Could you check a few things on this model? Use its own coordinates, in mm. A direction names the side the tool comes from. Coordinates: 2 decimals unless noted, no trailing zeros. Loops run counter-clockwise (first coordinate to the right, second up) from the corner with the lowest first, then second, coordinate; pieces in that order, holes last. Notation, with made-up numbers: (72, 25) -> (78, 25) arc R5 ccw to (78, 30) -> close; hole circle Ø2 at (42, 38). An arc over 180 degrees is marked (long way). One line per question, with ' | ' between items. Start each with the question number.
(1) Suppose I cut it at B-B (z = -14.5). Please give me the cut outline in (x, y).
(2) If we mould it in two halves opening along Z, with no side actions, what happens to faces 6 (the face through (0.27, -10.4, 43.93)), 7 (the face through (-12, -1, 26)), 8 (the face through (-9, 3.5, -45))? For each: pulls with the +Z half, pulls with the -Z half, needs draft (parallel to the pull), parting line crosses it, or undercut.
(3) Which directions (+Z, -Z, +X, -X, +Y, -Y) give clear straight access to the entire face, cutting with the end or side of a thin tool? Please do faces 1 (the face through (9.56, -6.07, 26.04)), 2 (the face through (-9, -1.5, -45)), 3 (the face through (0, 11, -1)), 4 (the face through (14.6, -7.2, -47)), 5 (the face through (-21, 0, 1)).
(4) Suppose I cut it at D-D (x = 1). Please give me the cut outline in (y, z), plus the area to 3 significant figures.
(5) Suppose I cut it at A-A (y = -6). Please give me the cut outline in (x, z), plus the area to 3 significant figures.
(6) If I drill on line 1 along X through (y, z) = (-6.5, 25.5); line 2 along X through (y, z) = (-7, -16.5); line 3 along Z through (x, y) = (-8, 8.75), over which ranges is the centre line in solid material (lowest first)?
(7) I'm going to push flat-ended pins straight in: pin 1 Ø4 at (x, y) = (-8, 0.5) entering from -Z; pin 2 Ø2.5 at (x, z) = (12, 25) entering from -Y; pin 3 Ø1 at (y, z) = (0, -45.5) entering from -X. Where does each tip first touch, or does it pass through?
(8) Suppose I cut it at C-C (y = 5). Please give me the cut outline in (x, z).
```python
from build123d import *

# Parameters (mm, degrees)
EXTRUDE_370_DEPTH      = 11
EXTRUDE_370_DEPTH_BACK = 11
SKETCH_1_W             = 42
SKETCH_1_H             = 89
SKETCH_2_W             = 7
SKETCH_2_H             = 5
EXTRUDE_597_DEPTH      = 2
SKETCH_3_R             = 2
EXTRUDE_827_DEPTH      = 5
SKETCH_4_R             = 2.5
CUT_EXTRUDE_1027_DEPTH = 10
FILLET_1_R             = 2


with BuildPart() as part:
    # Sketch 1 → Extrude 370 (new, two sides: drawn at the far end of the back side and taken through both)
    with BuildSketch(Plane(origin=(0, 0, 0), x_dir=(1, 0, 0), z_dir=(0, 1, 0)).offset(-EXTRUDE_370_DEPTH_BACK)):
        Rectangle(SKETCH_1_W, SKETCH_1_H)
    extrude(amount=EXTRUDE_370_DEPTH + EXTRUDE_370_DEPTH_BACK)

    # Sketch 2 → Extrude 597 (add)
    with BuildSketch(Plane(origin=(0, 0, -44.5), x_dir=(-1, 0, 0), z_dir=(0, 0, -1))):
        with Locations((9, 1)):
            Rectangle(SKETCH_2_W, SKETCH_2_H)
    extrude(amount=EXTRUDE_597_DEPTH)

    # Sketch 3 → Extrude 827 (add)
    with BuildSketch(Plane(origin=(0, 0, -44.5), x_dir=(-1, 0, 0), z_dir=(0, 0, -1))):
        with Locations((-13, -6)):
            Circle(SKETCH_3_R)
    extrude(amount=EXTRUDE_827_DEPTH)

    # Sketch 4 → Cut-Extrude 1027 (cut)
    with BuildSketch(Plane.XZ.offset(11)):
        with Locations(Location((-12, 25.5, 0), (0, 0, 270))):
            Circle(SKETCH_4_R)
        with Locations(Location((12, 25.5, 0), (0, 0, 270))):
            Circle(SKETCH_4_R)
        with Locations(Location((12, -14.5, 0), (0, 0, 270))):
            Circle(SKETCH_4_R)
        with Locations(Location((-12, -14.5, 0), (0, 0, 270))):
            Circle(SKETCH_4_R)
    extrude(amount=-CUT_EXTRUDE_1027_DEPTH, mode=Mode.SUBTRACT)

    # Fillet 1
    fillet_1_edges = [part.edges().sort_by_distance(p)[0] for p in [
        (-21, -11, 0),
        (21, 11, 0),
        (0, 11, -44.5),
        (0, -11, 44.5),
        (-21, 11, 0),
        (0, 11, 44.5),
        (21, -11, 0),
        (0, -11, -44.5),
        (21, 0, 44.5),
        (-21, 0, 44.5),
        (-21, 0, -44.5),
        (21, 0, -44.5),
    ]]
    fillet(fillet_1_edges, radius=FILLET_1_R)


solid = part.part
```
Checks:
1) outline: (-21, -9) arc R2 ccw to (-19, -11) -> (-14.5, -11) -> (-14.5, -1) -> (-9.5, -1) -> (-9.5, -11) -> (9.5, -11) -> (9.5, -1) -> (14.5, -1) -> (14.5, -11) -> (19, -11) arc R2 ccw to (21, -9) -> (21, 9) arc R2 ccw to (19, 11) -> (-19, 11) arc R2 ccw to (-21, 9) -> close
2) face 6: pulls with the +Z half | face 7: undercut | face 8: needs draft
3) face 1: -Y | face 2: -Z, +X, -X, -Y | face 3: +Z, -Z, +X, -X, +Y | face 4: -Z | face 5: +Z, -Z, -X, +Y, -Y
4) outline: (-11, -42.5) arc R2 ccw to (-9, -44.5) -> (9, -44.5) arc R2 ccw to (11, -42.5) -> (11, 42.5) arc R2 ccw to (9, 44.5) -> (-9, 44.5) arc R2 ccw to (-11, 42.5) -> close | area: 1,950 mm^2
5) outline: (-21, -42.5) arc R2 ccw to (-19, -44.5) -> (11, -44.5) -> (11, -49.5) -> (15, -49.5) -> (15, -44.5) -> (19, -44.5) arc R2 ccw to (21, -42.5) -> (21, 42.5) arc R2 ccw to (19, 44.5) -> (-19, 44.5) arc R2 ccw to (-21, 42.5) -> close; hole circle Ø5 at (-12, -14.5); hole circle Ø5 at (-12, 25.5); hole circle Ø5 at (12, -14.5); hole circle Ø5 at (12, 25.5) | area: 3,680 mm^2
6) line 1: x = -21 to -14.5, -9.5 to 9.5, 14.5 to 21 | line 2: x = -21 to -13.5, -10.5 to 10.5, 13.5 to 21 | line 3: z = -44.5 to 44.5
7) pin 1: stops at z = -46.5 | pin 2: stops at y = -1 | pin 3: stops at x = -12.5
8) outline: (-21, -42.5) arc R2 ccw to (-19, -44.5) -> (19, -44.5) arc R2 ccw to (21, -42.5) -> (21, 42.5) arc R2 ccw to (19, 44.5) -> (-19, 44.5) arc R2 ccw to (-21, 42.5) -> close
